Check sheet for the modelled part. Datum: model origin and axes. Units: mm. Face numbers are marked on the shaded views. Coordinates: 2 decimals unless noted, no trailing zeros. Order: outer loops, then holes, each group sorted by start corner. A loop starts at its lowest first (then second) coordinate and runs counter-clockwise, first axis right, second up.
1. Gauge pin test, flat ends, axial feed: pin 1 Ø13.5 at (x, z) = (0, -20) entering from +Y; pin 2 Ø4 at (x, z) = (0, 15) entering from +Y. Record the tip position at first contact, or that the pin passes through.
2. Cross-section at D-D (z = -22). Enter the section's corners in (x, y).
3. Cross-section at C-C (y = 4.7). Enter the section's corners in (x, z).
4. Cross-section at A-A (x = -6.5). Enter the section's corners in (y, z).
5. Cross-section at B-B (z = 0). Enter the section's corners in (x, y).
6. Draft check along X on the marked faces 1 and 2. Enter one of: released by +X, released by -X, zero draft, split by the parting line, or undercut.
7. Thickness scan on line 1 (Z direction, x = 0, y = 4.1); line 2 (Y direction, x = 12, z = -19); line 3 (X direction, y = 2.35, z = -15). Record the ranges inside material, lowest first.
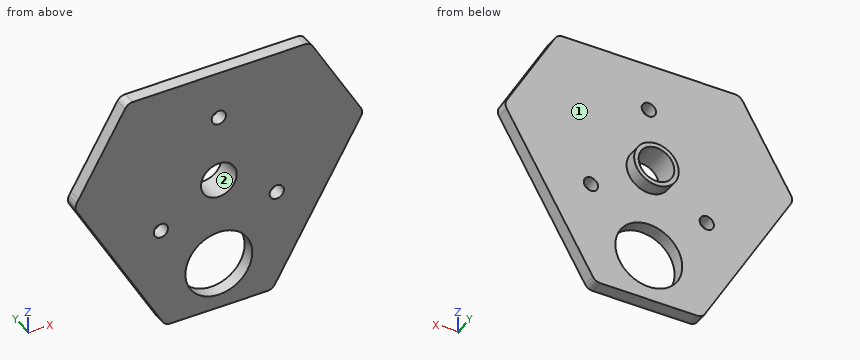
Autodesk Inventor part; units mm, degrees
ref_plane "YZ Plane" through (0, 0, 0) normal (1, 0, 0) x (0, 1, 0)
ref_plane "XZ Plane" through (0, 0, 0) normal (0, 1, 0) x (-1, 0, 0)
ref_plane "XY Plane" through (0, 0, 0) normal (0, 0, 1) x (1, 0, 0)
sketch "Sketch1" plane through (0, 0, 0) normal (0, 1, 0) x (-1, 0, 0)
  circle A0 centre (-12.9904, -7.5) radius 1.6
  circle A1 centre (12.9904, -7.5) radius 1.6
  circle A2 centre (0, 15) radius 1.6
  line L0 (31.4449, 6.6077) -> (21.0222, 24.6603)
  line L1 (10.8453, -30.5359) -> (-10.8453, -30.5359)
  line L2 (-21.0222, 24.6603) -> (-31.8675, 5.8756)
  line L3 (-31.8675, 3.8756) -> (-12.5774, -29.5359)
  line L4 (-19.2902, 25.6603) -> (19.2902, 25.6603)
  line L5 (20.4449, 25.6603) -> (31.8675, 5.8756)
  line L6 (31.8675, 3.8756) -> (12.5774, -29.5359)
  arc A3 (21.0222, 24.6603) -> (19.2902, 25.6603) centre (19.2902, 23.6603) ccw
  arc A4 (31.8675, 3.8756) -> (31.8675, 5.8756) centre (30.1355, 4.8756) ccw
  arc A5 (10.8453, -30.5359) -> (12.5774, -29.5359) centre (10.8453, -28.5359) ccw
  arc A6 (-12.5774, -29.5359) -> (-10.8453, -30.5359) centre (-10.8453, -28.5359) ccw
  arc A7 (-19.2902, 25.6603) -> (-21.0222, 24.6603) centre (-19.2902, 23.6603) ccw
  arc A8 (-31.8675, 5.8756) -> (-31.8675, 3.8756) centre (-30.1355, 4.8756) ccw
  circle A9 centre (0, 0) radius 4
  circle A10 centre (0, 0) radius 5
  dimension "d41" = 360
  dimension "d76" = 2
  dimension "d84" = 8
  dimension "d86" = 10
extrude "Extrusion8" add sketch "Sketch1" along normal blind 3 contours L5 A4 L6 A5 L1 A6 L3 A8 L2 A7 L4 A3 L0
extrude "Extrusion9" add sketch "Sketch1" along normal blind 6 contours A10
sketch "Sketch4" plane through (0, 3, 0) normal (0, 1, 0) x (1, 0, 0)
  point P0 (0, 0)
sketch "Sketch5" plane through (0, 3, 0) normal (0, 1, 0) x (1, 0, 0)
  circle A0 centre (0, 20) radius 7.5
  point P0 (0, 0)
  dimension "d91" = 15
extrude "Extrusion10" cut sketch "Sketch5" against normal blind 6
equation "\"BendRadius\" = Thickness"
equation "\"BendReliefWidth\" = Thickness"
equation "\"BendReliefDepth\" = 0.5 * Thickness"
equation "\"CornerReliefSize\" = 4 * Thickness"
equation "\"MinimumRemnant\" = 2 * Thickness"
equation "\"TransitionRadius\" = BendRadius"
equation "\"JacobiRadiusSize\" = BendRadius"
equation "\"GapSize\" = Thickness"
properties part number "Draw_Pen"
Data:
1. pin 1: passes through
1. pin 2: stops at y = 3
2. outline: (-16.93, 0) - (-7.23, 0) - (-7.23, 3) - (-16.93, 3) - close; (7.23, 0) - (16.93, 0) - (16.93, 3) - (7.23, 3) - close
3. outline: circle Ø10 at (0, 0); hole circle Ø8 at (0, 0)
4. outline: (0, -30.54) - (3, -30.54) - (3, -23.74) - (0, -23.74) - close; (0, -16.26) - (3, -16.26) - (3, 25.66) - (0, 25.66) - close
5. outline: (-29.63, 0) - (-4, 0) - (-4, 6) - (-5, 6) - (-5, 3) - (-29.63, 3) - close; (4, 0) - (29.63, 0) - (29.63, 3) - (5, 3) - (5, 6) - (4, 6) - close
6. face 1: zero draft
6. face 2: undercut
7. line 1: z = -5 to -4, 4 to 5
7. line 2: y = 0 to 3
7. line 3: x = -20.97 to -5.59, 5.59 to 20.97
